Autodesk Inventor part; units mm, degrees
ref_plane "作業平面4" through (16.7417, -2.952, 0) normal (0.9848, -0.1736, 0) x (0, 0, 1)
ref_plane "作業平面6" through (-16.7417, -2.952, 0) normal (0.9848, 0.1736, 0) x (0, 0, 1)
ref_plane "XZ Plane" through (0, 0, 0) normal (0, 1, 0) x (-1, 0, 0)
sketch "スケッチ1" plane through (0, 0, 0) normal (0, 0, 1) x (1, 0, 0)
  arc A0 (-17, 0) -> (17, 0) centre (0, 0) ccw
  arc A1 (-16, 0) -> (16, 0) centre (0, 0) ccw
  line L0 (-16, 0) -> (-17, 0)
  line L1 (16, 0) -> (17, 0)
  dimension "d0" = 17
  dimension "d66" = 1
extrude "押し出し1" add sketch "スケッチ1" along normal blind 45
ref_plane "作業平面4" through (16.7417, -2.952, 0) normal (0.9848, -0.1736, 0) x (0, 0, 1)
ref_plane "作業平面3" through (0, 0, 0) normal (0.9848, -0.1736, 0) x (0, 0, 1)
ref_plane "作業平面6" through (-16.7417, -2.952, 0) normal (0.9848, 0.1736, 0) x (0, 0, 1)
ref_plane "作業平面5" through (0, 0, 0) normal (0.9848, 0.1736, 0) x (0, 0, 1)
sketch "スケッチ8" plane through (16.7417, -2.952, 0) normal (0.9848, -0.1736, 0) x (0, 0, 1)
  line L0 (0, -5) -> (5, -5)
  line L1 (5, -5) -> (5, 5)
  line L2 (5, 5) -> (0, 5)
  line L3 (0, 5) -> (0, -5)
  line L4 (0, 0) -> (8.4852, 0) construction
  dimension "d38" = 5
  dimension "d39" = 10
extrude "押し出し8" cut sketch "スケッチ8" against normal blind 0.5
sketch "スケッチ9" plane through (-16.7417, -2.952, 0) normal (0.9848, 0.1736, 0) x (0, 0, 1)
  line L0 (0, -5) -> (5, -5)
  line L1 (5, -5) -> (5, 5)
  line L2 (5, 5) -> (0, 5)
  line L3 (0, 5) -> (0, -5)
  line L4 (0, 0) -> (8.3316, 0) construction
  dimension "d42" = 5
  dimension "d43" = 10
extrude "押し出し9" cut sketch "スケッチ9" along normal blind 0.5
sketch "スケッチ11" plane through (16.2493, -2.8652, 0) normal (0.9848, -0.1736, 0) x (0, 0, -1)
  circle A0 centre (-2.5, 0) radius 1.2
  point P0 (0, 0)
  dimension "d50" = 2.4
  dimension "d51" = 2.5
extrude "押し出し11" cut sketch "スケッチ11" against normal blind 1
sketch "スケッチ12" plane through (-16.2493, -2.8652, 0) normal (-0.9848, -0.1736, 0) x (0, 0, 1)
  circle A0 centre (2.5, 0) radius 1.2
  point P0 (0, 0)
  dimension "d54" = 2.4
  dimension "d55" = 2.5
extrude "押し出し12" cut sketch "スケッチ12" against normal blind 1
properties part number "B_shield_5" material "ステンレス鋼 440C"
Build history of the part. All positions in model axes, mm. A direction names the side the tool comes from. Round coordinates to 2 decimals unless told otherwise and drop trailing zeros. Loops run counter-clockwise (first coordinate to the right, second up) from the corner with the lowest first, then second, coordinate; pieces in that order, holes last. Notation, with made-up numbers: (0.25, -30) -> (20.25, -30) arc R33 cw to (20.25, -2) -> close; hole circle Ø2 at (36.5, 80). An arc over 180 degrees is marked (long way). Answer in a Markdown table with one row per item.
Item 1: Drill centre lines: L1, parallel to X at y = -0.5, z = 21.5; L2, parallel to X at y = -14.75, z = 16; L3, parallel to Y at x = -6.5, z = 32.5. Where is each one in solid material? Low to high. Write a range as [from, to].
Answers below:
| item | result |
|---|---|
| L1 | x = [-16.99, -15.99], [15.99, 16.99] |
| L2 | x = [-8.45, -6.2], [6.2, 8.45] |
| L3 | y = [-15.71, -14.62] |
Item 2: Pin check, flat tips, straight feed: pin 1 (6 mm diameter, centred on y = -4, z = 16.5, fed in from +X); pin 2 (3 mm diameter, centred on x = 9, z = 18.5, fed in from -Y); pin 3 (12 mm diameter, centred on x = 8, z = 15.5, fed in from -Y). Stop position of each tip, or through.
Answers below:
| item | result |
|---|---|
| pin 1 | stops at x = 16.97 |
| pin 2 | stops at y = -15.26 |
| pin 3 | stops at y = -16.88 |
Item 3: Saw through at B-B (x = 0). Write the cut outline in (y, z).
Answers below:
| item | result |
|---|---|
| outline | (-17, 0) -> (-16, 0) -> (-16, 45) -> (-17, 45) -> close |
Item 4: Mould opens along Y. For faces 1 (the cylindrical face through (0, -17, 22)), 2 (the cylindrical face through (0, -16, 22)), 3 (the cylindrical face through (-16, -2.8, 1.3)) say: +Y half, -Y half, draft (parallel to the pull), parting line (faces both ways), or undercut.
Answers below:
| item | result |
|---|---|
| face 1 | -Y half |
| face 2 | +Y half |
| face 3 | undercut |
Item 5: Saw through at C-C (z = 14.5). Write the cut outline in (x, y), and give its area (3 significant figures).
Answers below:
| item | result |
|---|---|
| outline | (-17, 0) arc R17 ccw to (17, 0) -> (16, 0) arc R16 cw to (-16, 0) -> close |
| area | 51.8 mm² |
Item 6: Saw through at A-A (y = -13). Write the cut outline in (x, z), and give its area (3 significant figures).
Answers below:
| item | result |
|---|---|
| outline | (-10.95, 0) -> (-9.33, 0) -> (-9.33, 45) -> (-10.95, 45) -> close; (9.33, 0) -> (10.95, 0) -> (10.95, 45) -> (9.33, 45) -> close |
| area | 146 mm² |
Item 7: Saw through at D-D (y = -9). Write the cut outline in (x, z), and give its area (3 significant figures).
Answers below:
| item | result |
|---|---|
| outline | (-14.42, 0) -> (-13.23, 0) -> (-13.23, 45) -> (-14.42, 45) -> close; (13.23, 0) -> (14.42, 0) -> (14.42, 45) -> (13.23, 45) -> close |
| area | 107 mm² |
Item 8: Which spindle directions (+Z, -Z, +X, -X, +Y, -Y) get a long thin tool onto all of the face, cutting with end or side? Do faces 4 (the flat face through (-16, -4.27, 2.47)), 5 (the flat face through (16.4, -3.4, 5)), 6 (the flat face through (-16.5, 0, 22.2)). Say none if no direction does.
Answers below:
| item | result |
|---|---|
| face 4 | -Z, -X, -Y |
| face 5 | -Z, +X, -Y |
| face 6 | +Z, -Z, +X, -X, +Y |
